Could you check a few things on this model? Use its own coordinates, in mm. Face numbers are marked on the shaded views. Give positions to 0.01 mm unless a question says otherwise; leave off trailing zeros. Loops run counter-clockwise (first coordinate to the right, second up) from the corner with the lowest first, then second, coordinate; pieces in that order, holes last. Notation, with made-up numbers: (49.25, -18.75) -> (94.25, -18.75) arc R25 ccw to (94.25, 8.25) -> close; hole circle Ø8 at (87, 45.5). An arc over 180 degrees is marked (long way). Write each question's results on one line, items separated by ' | '. Start each with the question number.
Q1. If I drill on line 1 along X through (y, z) = (9, 0); line 2 along X through (y, z) = (4, 0); line 3 along Z through (x, y) = (-22, 2), over which ranges is the centre line in solid material (lowest first)?
Q2. If we section it at B-B, the plane z = 0: List the corners of the cut face in (x, y) for me, plus the area to 4 significant figures.
Q3. If we section it at D-D, the plane z = 32: List the corners of the cut face in (x, y) for me, plus the area to 3 significant figures.
Q4. Will these pins go through, and if not, where does the flat tip stop? P1, Ø1, axis at y = -5.5, z = -18, coming from the +X side; P2, Ø1, axis at x = 32, y = -11.5, coming from the +Z side; P3, Ø5, axis at y = -6.5, z = 14.5, coming from the +X side.
Q5. We'd pull the mould along Z, two halves only. Please class the marked faces 1, 2 and 3: released by +Z, released by -Z, zero draft, split by the parting line, or undercut.
Q6. If we section it at A-A, the plane x = 0: List the corners of the cut face in (y, z) for me, plus the area to 4 significant figures.
Q7. If we section it at C-C, the plane y = 5: List the corners of the cut face in (x, z) for me, plus the area to 3 significant figures.
from build123d import *

# Parameters (mm, degrees)
SKETCH1_R           = 47.5
SKETCH1_R_2         = 25
BOSS_EXTRUDE1_DEPTH = 15.5
SKETCH3_R           = 47.5
SKETCH3_R_2         = 45
CUT_EXTRUDE1_DEPTH  = 8


with BuildPart() as part:
    # Sketch1 → Boss-Extrude1 (new, symmetric)
    with BuildSketch(Plane(origin=(0, 0, 0), x_dir=(1, 0, 0), z_dir=(0, 1, 0))):
        with Locations(Location((0, 0, 0), (0, 0, 270))):
            Circle(SKETCH1_R)
        with Locations(Location((0, 0, 0), (0, 0, 270))):
            Circle(SKETCH1_R_2, mode=Mode.SUBTRACT)
    extrude(amount=BOSS_EXTRUDE1_DEPTH, both=True)

    # Sketch3 → Cut-Extrude1 (cut, symmetric)
    with BuildSketch(Plane(origin=(0, 0, 0), x_dir=(1, 0, 0), z_dir=(0, 1, 0))):
        with Locations(Location((0, 0, 0), (0, 0, 270))):
            Circle(SKETCH3_R)
        with Locations(Location((0, 0, 0), (0, 0, 270))):
            Circle(SKETCH3_R_2, mode=Mode.SUBTRACT)
    extrude(amount=CUT_EXTRUDE1_DEPTH, both=True, mode=Mode.SUBTRACT)


solid = part.part
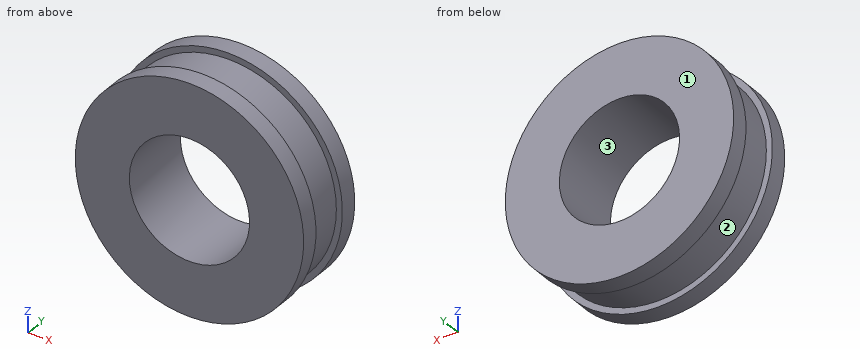
Final values:
1) line 1: x = -47.5 to -25, 25 to 47.5 | line 2: x = -45 to -25, 25 to 45 | line 3: z = -39.26 to -11.87, 11.87 to 39.26
2) outline: (-47.5, -15.5) -> (-25, -15.5) -> (-25, 15.5) -> (-47.5, 15.5) -> (-47.5, 8) -> (-45, 8) -> (-45, -8) -> (-47.5, -8) -> close; (25, -15.5) -> (47.5, -15.5) -> (47.5, -8) -> (45, -8) -> (45, 8) -> (47.5, 8) -> (47.5, 15.5) -> (25, 15.5) -> close | area: 1,315 mm²
3) outline: (-35.1, -15.5) -> (35.1, -15.5) -> (35.1, -8) -> (31.64, -8) -> (31.64, 8) -> (35.1, 8) -> (35.1, 15.5) -> (-35.1, 15.5) -> (-35.1, 8) -> (-31.64, 8) -> (-31.64, -8) -> (-35.1, -8) -> close | area: 2,070 mm²
4) P1: stops at x = 41.46 | P2: stops at z = 35.55 | P3: stops at x = 45.83
5) face 1: zero draft | face 2: split by the parting line | face 3: undercut
6) outline: (-15.5, -47.5) -> (-8, -47.5) -> (-8, -45) -> (8, -45) -> (8, -47.5) -> (15.5, -47.5) -> (15.5, -25) -> (-15.5, -25) -> close; (-15.5, 25) -> (15.5, 25) -> (15.5, 47.5) -> (8, 47.5) -> (8, 45) -> (-8, 45) -> (-8, 47.5) -> (-15.5, 47.5) -> close | area: 1,315 mm²
7) outline: circle Ø90 at (0, 0); hole circle Ø50 at (0, 0) | area: 4,400 mm²
